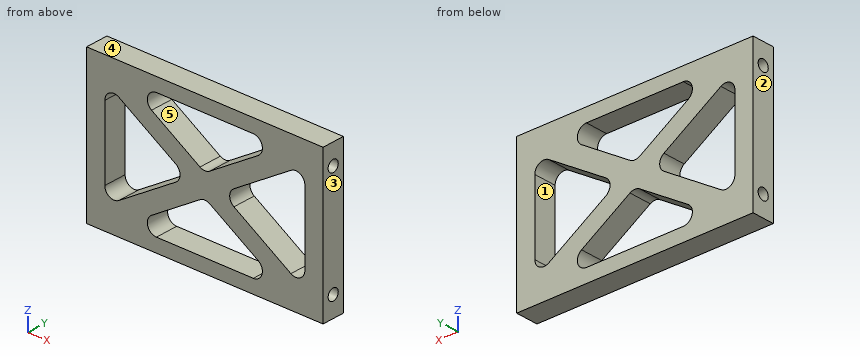
```python
from build123d import *

# Parameters (mm, degrees)
SKETCH1_W           = 52
SKETCH1_H           = 33
BOSS_EXTRUDE1_DEPTH = 5
FILLET1_R           = 2
SKETCH2_R           = 1.25
CUT_EXTRUDE1_DEPTH  = 12


with BuildPart() as part:
    # Sketch1 → Boss-Extrude1 (new body)
    with BuildSketch(Plane(origin=(0, 0, 0), x_dir=(1, 0, 0), z_dir=(0, 1, 0))):
        with Locations((26, 16.5)):
            Rectangle(SKETCH1_W, SKETCH1_H)
        Polygon((4, 28.092794755), (4, 4.907205245), (22.26743416, 16.5), align=None, mode=Mode.SUBTRACT)
        Polygon((26, 14.131256294), (8.459838567, 3), (43.540161433, 3), align=None, mode=Mode.SUBTRACT)
        Polygon((48, 4.907205245), (29.73256584, 16.5), (48, 28.092794755), align=None, mode=Mode.SUBTRACT)
        Polygon((8.459838567, 30), (43.540161433, 30), (26, 18.868743706), align=None, mode=Mode.SUBTRACT)
    extrude(amount=BOSS_EXTRUDE1_DEPTH)

    # Fillet1
    fillet1_edges = [part.edges().sort_by_distance(p)[0] for p in [
        (22.26743416, 2.5, -16.5),
        (4, 2.5, -28.092794755),
        (4, 2.5, -4.907205245),
        (43.540161433, 2.5, -3),
        (26, 2.5, -14.131256294),
        (8.459838567, 2.5, -3),
        (48, 2.5, -4.907205245),
        (48, 2.5, -28.092794755),
        (29.73256584, 2.5, -16.5),
        (8.459838567, 2.5, -30),
        (26, 2.5, -18.868743706),
        (43.540161433, 2.5, -30),
    ]]
    fillet(fillet1_edges, radius=FILLET1_R)

    # Sketch2 → Cut-Extrude1 (cut)
    with BuildSketch(Plane(origin=(52, 0, 0), x_dir=(0, 0, -1), z_dir=(1, 0, 0))):
        with Locations((4.5, 2.5)):
            Circle(SKETCH2_R)
        with Locations(Location((28.5, 2.5, 0), (0, 0, 180))):
            Circle(SKETCH2_R)
    cut_extrude1 = extrude(amount=-CUT_EXTRUDE1_DEPTH, mode=Mode.SUBTRACT)

    # Mirror1: Cut-Extrude1 across plane
    add(cut_extrude1.mirror(Plane(origin=(26, 0, 0), x_dir=(0, 0, 1), z_dir=(1, 0, 0))), mode=Mode.SUBTRACT)


solid = part.part
```
Geometry check sheet. Reference: the model listing, model coordinates, mm. Face numbers are marked on the shaded views. A direction names the side the tool comes from. Coordinates: 2 decimals unless noted, no trailing zeros. Write each loop counter-clockwise with the first axis right and the second up, starting at its lowest first coordinate (ties: lowest second). Pieces come first, ordered by that corner, then holes. Notation, with made-up numbers: M 31.25,-18.75 L 45.25,-18.75 A17 ccw 45.25,7.25 Z; hole C 12.25,58 d9. An arc over 180 degrees is marked long. Answer as a JSON object with one key per item and string values.
1. Section check B-B, the plane x = 18. Enter the section's corners in (y, z).
Answers below:
{"outline": "M 0,-33 L 5,-33 L 5,-30 L 0,-30 Z; M 0,-23.95 L 5,-23.95 L 5,-19.21 L 0,-19.21 Z; M 0,-13.79 L 5,-13.79 L 5,-9.05 L 0,-9.05 Z; M 0,-3 L 5,-3 L 5,0 L 0,0 Z"}
2. Go/stop test with flat-tipped pins: pin 1 Ø2 at (y, z) = (2.5, -28.5) entering from -X; pin 2 Ø2 at (y, z) = (2.5, -4.5) entering from +X. Record where each tip stops, or that it passes through.
Answers below:
{"pin 1": "stops at x = 12", "pin 2": "stops at x = 40"}
3. Tool access check on the marked faces 1 and 2. Record the directions out of +Z, -Z, +X, -X, +Y, -Y that give a thin tool (end or side, any length) a straight path to the whole face; none if there is none.
Answers below:
{"face 1": "+Y, -Y", "face 2": "+Z, -Z, -X, +Y, -Y"}
4. Draft check along X on the marked faces 3, 4 and 5. Enter one of: released by +X, released by -X, zero draft, split by the parting line, or undercut.
Answers below:
{"face 3": "released by +X", "face 4": "zero draft", "face 5": "undercut"}
5. Section check C-C, the plane z = -10. Enter the section's corners in (x, y) (3 decimals), plus the area to 3 significant figures.
Answers below:
{"outline": "M 0,0 L 4,0 L 4,5 L 0,5 Z; M 12.025,0 L 19.49,0 L 19.49,5 L 12.025,5 Z; M 32.51,0 L 39.975,0 L 39.975,5 L 32.51,5 Z; M 48,0 L 52,0 L 52,5 L 48,5 Z", "area": "115 mm²"}
6. Scan lines: L1, parallel to Y at x = 47.25, z = -28.5; L2, parallel to X at y = 3, z = -13; L3, parallel to X at y = 4.2, z = -12. Record each from-to range of solid material in increasing order.
Answers below:
{"L1": "y = 0 to 1.25, 3.75 to 5", "L2": "x = 0 to 4, 16.75 to 24.22, 27.78 to 35.25, 48 to 52", "L3": "x = 0 to 4, 15.18 to 22.64, 29.36 to 36.82, 48 to 52"}
7. Section check A-A, the plane y = 0.65. Enter the section's corners in (x, z), plus the area to 3 significant figures.
Answers below:
{"outline": "M 0,-33 L 52,-33 L 52,0 L 0,0 Z; hole M 4,-24.45 A2 ccw 7.07,-26.14 L 19.61,-18.19 A2 ccw 19.61,-14.81 L 7.07,-6.86 A2 ccw 4,-8.55 Z; hole M 14.27,-26.31 A2 ccw 15.34,-30 L 36.66,-30 A2 ccw 37.73,-26.31 L 27.07,-19.55 A2 ccw 24.93,-19.55 Z; hole M 14.27,-6.69 L 24.93,-13.45 A2 ccw 27.07,-13.45 L 37.73,-6.69 A2 ccw 36.66,-3 L 15.34,-3 A2 ccw Z; hole M 32.39,-18.19 L 44.93,-26.14 A2 ccw 48,-24.45 L 48,-8.55 A2 ccw 44.93,-6.86 L 32.39,-14.81 A2 ccw Z", "area": "954 mm²"}
8. Section check D-D, the plane x = 29. Enter the section's corners in (y, z), plus the area to 3 significant figures.
Answers below:
{"outline": "M 0,-33 L 5,-33 L 5,-30 L 0,-30 Z; M 0,-20.77 L 5,-20.77 L 5,-12.23 L 0,-12.23 Z; M 0,-3 L 5,-3 L 5,0 L 0,0 Z", "area": "72.7 mm²"}
